Could you check a few things on this model? Use its own coordinates, in mm. Coordinates: 2 decimals unless noted, no trailing zeros. Answer as a JSON object with one key per item and string values. Group by question number.
(1) Will this pin go through, and if not, where does the flat tip stop? P1, Ø5, axis at x = 0, y = 50, coming from the -Z side.
(2) We'd pull the mould along Y, two halves only. Please class faces 1 (the flat face through (-2, 20, 0)), 2 (the cylindrical face through (-17.669, -15.163, 2.465)): pulls with the +Y half, pulls with the -Y half, needs draft (parallel to the pull), parting line crosses it, or undercut.
(3) Please list where these lines run through material, in increasing order: probe 1 along Y at (x, z) = (100, 2.05); probe 2 along X at (y, z) = (-2, 3.2).
from build123d import *

# Parameters (mm, degrees)
SKETCH_1_W          = 300
SKETCH_1_H          = 250
SKETCH_1_R          = 3.3
SKETCH_1_R_2        = 2.5
EXTRUDE_1_DEPTH     = 5
SKETCH_2_R          = 2.75
CUT_EXTRUDE_1_DEPTH = 196.320249846
SKETCH_3_W          = 300
SKETCH_3_H          = 40
CUT_EXTRUDE_2_DEPTH = 196.320249846


with BuildPart() as part:
    # 草图1 → 凸台-拉伸1 (new body)
    with BuildSketch(Plane.XY):
        Rectangle(SKETCH_1_W, SKETCH_1_H)
        with Locations((-18.384776311, 18.384776311)):
            Circle(SKETCH_1_R, mode=Mode.SUBTRACT)
        with Locations(Location((18.384776311, 18.384776311, 0), (0, 0, 180))):
            Circle(SKETCH_1_R, mode=Mode.SUBTRACT)
        with Locations((18.384776311, -18.384776311)):
            Circle(SKETCH_1_R, mode=Mode.SUBTRACT)
        with Locations(Location((-18.384776311, -18.384776311, 0), (0, 0, 180))):
            Circle(SKETCH_1_R, mode=Mode.SUBTRACT)
        Circle(SKETCH_1_R_2, mode=Mode.SUBTRACT)
    extrude(amount=EXTRUDE_1_DEPTH)

    # 草图2 → 切除-拉伸1 (cut, through all)
    with BuildSketch(Plane.XY.offset(5)):
        with Locations((-100, 50)):
            Circle(SKETCH_2_R)
        with Locations((0, 50)):
            Circle(SKETCH_2_R)
        with Locations((100, 50)):
            Circle(SKETCH_2_R)
        with Locations((100, -50)):
            Circle(SKETCH_2_R)
        with Locations((0, -50)):
            Circle(SKETCH_2_R)
        with Locations((-100, -50)):
            Circle(SKETCH_2_R)
    extrude(amount=-CUT_EXTRUDE_1_DEPTH, mode=Mode.SUBTRACT)

    # 草图3 → 切除-拉伸2 (cut, through all)
    with BuildSketch(Plane.XY.offset(5)):
        with Locations((0, 105)):
            Rectangle(SKETCH_3_W, SKETCH_3_H)
        with Locations((0, -105)):
            Rectangle(SKETCH_3_W, SKETCH_3_H)
    extrude(amount=-CUT_EXTRUDE_2_DEPTH, mode=Mode.SUBTRACT)


solid = part.part
Result set:
{
 "1": {"P1": "passes through"},
 "2": {"face 1": "needs draft", "face 2": "undercut"},
 "3": {"probe 1": "y = -85 to -52.75, -47.25 to 47.25, 52.75 to 85", "probe 2": "x = -150 to -1.5, 1.5 to 150"}
}
